```python
from build123d import *

# Parameters (mm, degrees)
F0_R     = 5.5
F1_DEPTH = 2.5
F3_DEPTH = 4
F4_R     = 1
F5_DEPTH = 50
F6_R     = 2.5
F7_DEPTH = 4


with BuildPart() as f1:
    # F0 (on Top) → F1 (new body, symmetric)
    with BuildSketch(Plane.XY):
        Circle(F0_R)
    extrude(amount=F1_DEPTH, both=True)

    # F2 (on Top) → F3 (join)
    with BuildSketch(Plane.XY):
        Polygon((-2.5, -1.443376), (0, -2.886751), (2.5, -1.443376), (2.5, 1.443376), (0, 2.886751), (-2.5, 1.443376), align=None)
    extrude(amount=F3_DEPTH)

    # F4 (on Right) → F5 (cut, symmetric)
    with BuildSketch(Plane.YZ):
        with Locations((0, -0.5)):
            Circle(F4_R)
    extrude(amount=F5_DEPTH, both=True, mode=Mode.SUBTRACT)

    # F6 (on face) → F7 (cut)
    with BuildSketch(Plane(origin=(0, 0, -2.5), x_dir=(1, 0, 0), z_dir=(0, 0, -1))):
        Circle(F6_R)
    extrude(amount=-F7_DEPTH, mode=Mode.SUBTRACT)


solid = f1.part
```
The listing builds one solid part. Answer for the finished solid, in the listing's coordinates (mm). A direction names the side the tool comes from. Round coordinates to 2 decimals unless told otherwise and drop trailing zeros. Order: outer loops, then holes, each group sorted by start corner. A loop starts at its lowest first (then second) coordinate and runs counter-clockwise, first axis right, second up. Notation, with made-up numbers: (-20, 79.5) -> (12, 79.5) arc R12 cw to (12, 91.5) -> close; hole circle Ø5 at (15.5, -3). An arc over 180 degrees is marked (long way). Answer as CSV lines item,"result".
Q1. A cutting plane is placed at D-D on x = -2. Determine the outline of the cut face in (y, z), plus the area to 3 significant figures.
Computed values:
outline,"(-5.12, -2.5) -> (-1.5, -2.5) -> (-1.5, 1.5) -> (1.5, 1.5) -> (1.5, -2.5) -> (5.12, -2.5) -> (5.12, 2.5) -> (1.73, 2.5) -> (1.73, 4) -> (-1.73, 4) -> (-1.73, 2.5) -> (-5.12, 2.5) -> close"
area,"44.4 mm^2"
Q2. Which of the six approach directions +Z, -Z, +X, -X, +Y, -Y give full straight-line access (tool end or side, diameter ignored) to faces 4 (the flat face through (-1.267, -2.155, 3.24)), 5 (the flat face through (-2.5, 0, 3)), 6 (the flat face through (0, 0, 1.5))?
Computed values:
face 4,"+Z, -X, -Y"
face 5,"+Z, -X, +Y, -Y"
face 6,"-Z"
Q3. A cutting plane is placed at B-B on z = -0.5. Determine the outline of the cut face in (x, y), plus the area to 3 significant figures.
Computed values:
outline,"(-5.41, -1) arc R5.5 ccw to (5.41, -1) -> (2.29, -1) arc R2.5 cw to (-2.29, -1) -> close; (-5.41, 1) -> (-2.29, 1) arc R2.5 cw to (2.29, 1) -> (5.41, 1) arc R5.5 ccw to start"
area,"63.2 mm^2"
Q4. Given pin 1 (1.2 mm diameter, centred on y = 0.5, z = 3.5, fed in from +X), flat-ended and moving along its own axis, determine where the tip first touches the part or whether it passes through.
Computed values:
pin 1,"stops at x = 2.5"
Q5. A cutting plane is placed at A-A on y = 0. Determine the outline of the cut face in (x, z), plus the area to 3 significant figures.
Computed values:
outline,"(-5.5, -2.5) -> (-2.5, -2.5) -> (-2.5, -1.5) -> (-5.5, -1.5) -> close; (-5.5, 0.5) -> (-2.5, 0.5) -> (-2.5, 1.5) -> (2.5, 1.5) -> (2.5, 0.5) -> (5.5, 0.5) -> (5.5, 2.5) -> (2.5, 2.5) -> (2.5, 4) -> (-2.5, 4) -> (-2.5, 2.5) -> (-5.5, 2.5) -> close; (2.5, -2.5) -> (5.5, -2.5) -> (5.5, -1.5) -> (2.5, -1.5) -> close"
area,"30.5 mm^2"
Q6. A cutting plane is placed at C-C on x = -4. Determine the outline of the cut face in (y, z), plus the area to 3 significant figures.
Computed values:
outline,"(-3.77, -2.5) -> (3.77, -2.5) -> (3.77, 2.5) -> (-3.77, 2.5) -> close; hole circle Ø2 at (0, -0.5)"
area,"34.6 mm^2"
Q7. For a pull along Y with two mould halves and no side action, classify faces 1 (the cylindrical face through (1.15, 2.22, -0.53)), 2 (the flat face through (-1.233, 2.175, 3.24)), 3 (the flat face through (2.5, 0, 3)) as +Y half, -Y half, draft (parallel to the pull), parting line (faces both ways), or undercut.
Computed values:
face 1,"undercut"
face 2,"+Y half"
face 3,"draft"
Q8. Consider line 1 (Z direction, x = -3.2, y = 0); line 2 (X direction, y = 0, z = 0.55); line 3 (Y direction, x = 5, z = 2). Determine where each line is inside the solid, lowest interval first. Write a range as from..to.
Computed values:
line 1,"z = -2.5..-1.5, 0.5..2.5"
line 2,"x = -5.5..-2.5, 2.5..5.5"
line 3,"y = -2.29..2.29"
